```python
from build123d import *

# Parameters (mm, degrees)
FILLET2_R = 3


with BuildPart() as part:
    # Sketch1 → Revolve1 (revolve)
    with BuildSketch(Plane.XY, mode=Mode.PRIVATE) as revolve1_sk:
        Polygon((9, 60), (4, 60), (4, 45), (-4, 45), (-4, 15), (-9, 15), (-9, 12), (-1, 12), (-1, 42), (7, 42), (7, 55), (9, 55), align=None)
    revolve(revolve1_sk.sketch.rotate(Axis((-9, 0, 0), (1, 0, 0)), 90), axis=Axis((-9, 0, 0), (1, 0, 0)))

    # Fillet2
    fillet2_edges = [part.edges().sort_by_distance(p)[0] for p in [
        (-9, 0, -15),
        (-4, 0, -45),
        (4, 0, -60),
    ]]
    fillet(fillet2_edges, radius=FILLET2_R - 0.0001)  # a hair under: the kernel refuses the full size


solid = part.part
```
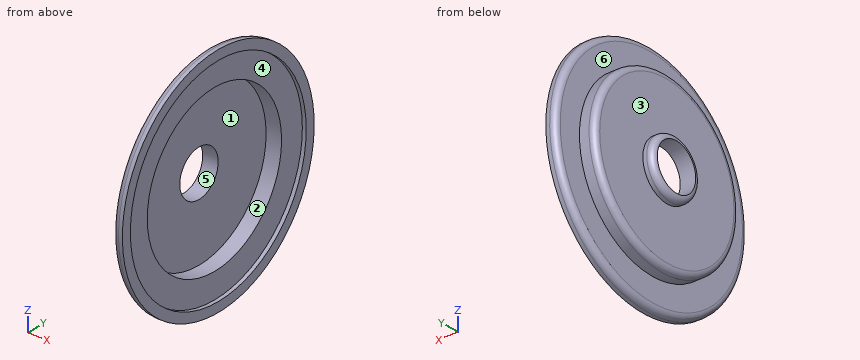
Here's how the part is built. I have some questions about the finished solid (model axes, mm). Face numbers are marked on the shaded views. A direction names the side the tool comes from. Coordinates: 2 decimals unless noted, no trailing zeros. Loops run counter-clockwise (first coordinate to the right, second up) from the corner with the lowest first, then second, coordinate; pieces in that order, holes last. Notation, with made-up numbers: M -3,-39.5 L 41,-39.5 A22 ccw 41,-27.5 Z; hole C -3,73 d11. An arc over 180 degrees is marked long. One line per item, written item: value.
1. Thinking about a two-plate mould opening in Z: for the marked faces 1, 2 and 3, which applies, +Z half, -Z half, draft (parallel to the pull), parting line (faces both ways), or undercut?
Geometry says:
face 1: undercut
face 2: undercut
face 3: draft
2. Imagine slicing it at C-C (x = 0.75). List the corners of the cut face in (y, z) for me.
Geometry says:
outline: C 0,0 d90; hole C 0,0 d84
3. Please list where these lines run through material, in increasing order: probe 1 along Y at (x, z) = (-5.25, 0); probe 2 along Y at (x, z) = (1.25, 0); probe 3 along X at (y, z) = (-11, -49.5).
Geometry says:
probe 1: y = -15 to -12, 12 to 15
probe 2: y = -45 to -42, 42 to 45
probe 3: x = 4 to 7
4. On a 3-axis mill with a long thin cutter (end or side, diameter ignored), from which of +Z, -Z, +X, -X, +Y, -Y can I reach the whole of each face in a straight line? I mean the marked faces 4, 5 and 6. Say none if no direction works.
Geometry says:
face 4: +X
face 5: +X, -X
face 6: -X
5. Will these pins go through, and if not, where does the flat tip stop? pin 1 Ø4 at (x, y) = (7, 6.5) entering from +Z; pin 2 Ø3 at (x, y) = (4.5, 18) entering from -Z; pin 3 Ø5 at (y, z) = (-17, -1) entering from -X.
Geometry says:
pin 1: stops at z = 59.83
pin 2: stops at z = -57.21
pin 3: stops at x = -7.61
